from build123d import *

# Parameters (mm, degrees)
SKETCH1_R           = 15
SKETCH1_R_2         = 10
BOSS_EXTRUDE1_DEPTH = 125
SKETCH2_R           = 15
BOSS_EXTRUDE2_DEPTH = 40
SKETCH6_W           = 20
SKETCH6_H           = 5
BOSS_EXTRUDE6_DEPTH = 100
FILLET1_R           = 10
SKETCH8_W           = 28
SKETCH8_H           = 2
BOSS_EXTRUDE7_DEPTH = 30
CUT_EXTRUDE1_DEPTH  = 30
SKETCH10_R          = 6.25
CUT_EXTRUDE2_DEPTH  = 30


with BuildPart() as part:
    # Sketch1 → Boss-Extrude1 (new body)
    with BuildSketch(Plane(origin=(0, 0, 0), x_dir=(1, 0, 0), z_dir=(0, 1, 0))):
        with Locations(Location((0, 0, 0), (0, 0, 270))):
            Circle(SKETCH1_R)
        with Locations(Location((0, 0, 0), (0, 0, 270))):
            Circle(SKETCH1_R_2, mode=Mode.SUBTRACT)
    extrude(amount=BOSS_EXTRUDE1_DEPTH)

    # Sketch2 → Boss-Extrude2 (add)
    with BuildSketch(Plane.XY):
        with Locations((0, 62.5)):
            Circle(SKETCH2_R)
    extrude(amount=BOSS_EXTRUDE2_DEPTH)

    # Sketch6 → Boss-Extrude6 (add)
    with BuildSketch(Plane(origin=(0, 0, 0), x_dir=(0, 0, -1), z_dir=(1, 0, 0))):
        with Locations((0, 62.5)):
            Rectangle(SKETCH6_W, SKETCH6_H)
    extrude(amount=BOSS_EXTRUDE6_DEPTH)

    # Fillet1
    fillet1_edges = [part.edges().sort_by_distance(p)[0] for p in [
        (100, 62.5, -10),
        (100, 62.5, 10),
    ]]
    fillet(fillet1_edges, radius=FILLET1_R - 0.0001)  # a hair under: the kernel refuses the full size

    # Sketch8 → Boss-Extrude7 (add)
    with BuildSketch(Plane(origin=(0, 65, 0), x_dir=(1, 0, 0), z_dir=(0, 1, 0))):
        with Locations((28.5, 0)):
            Rectangle(SKETCH8_W, SKETCH8_H)
    extrude(amount=BOSS_EXTRUDE7_DEPTH)

    # Sketch9 → Cut-Extrude1 (cut)
    with BuildSketch(Plane(origin=(0, 0, -1), x_dir=(-1, 0, 0), z_dir=(0, 0, -1))):
        Polygon((-14.966629547, 95), (-42.5, 65), (-42.5, 95), align=None)
    extrude(amount=-CUT_EXTRUDE1_DEPTH, mode=Mode.SUBTRACT)

    # Sketch10 → Cut-Extrude2 (cut)
    with BuildSketch(Plane(origin=(0, 65, 0), x_dir=(1, 0, 0), z_dir=(0, 1, 0))):
        with Locations(Location((90, 0, 0), (0, 0, 270))):
            Circle(SKETCH10_R)
    extrude(amount=-CUT_EXTRUDE2_DEPTH, mode=Mode.SUBTRACT)


solid = part.part
Read the model definition and answer for the solid it produces. Units are mm, in the model's axes. A direction names the side the tool comes from. Give positions to 0.01 mm unless a question says otherwise; leave off trailing zeros. Write each loop counter-clockwise with the first axis right and the second up, starting at its lowest first coordinate (ties: lowest second). Pieces come first, ordered by that corner, then holes. Notation, with made-up numbers: (50.5, 22) - (108.5, 22) arc R27 ccw to (108.5, 56) - close; hole circle Ø4 at (6.5, -0.75). An arc over 180 degrees is marked (long way). Use CSV: the item, a comma, the result in double quotes. Start each with the question number.
Item 1: The part is cut by section B-B, the plane x = -8. Give the vertices of the cut face in (y, z).
Item 2: For faces 4 (the flat face through (4, 60, -4)), 5 (the flat face through (25, 76, 1)), 6 (the flat face through (55, 65, 0)), 7 (the cylindrical face through (-14.985, 63.16, 24.164)), determine the directions among +Z, -Z, +X, -X, +Y, -Y from which every point of the face is accessible in a straight line to the end or side of a thin tool.
Item 3: The part is cut by section D-D, the plane y = 97.5. Give the vertices of the cut face in (x, z).
Item 4: Consider line 1 (X direction, y = 37.5, z = 0); line 2 (Y direction, x = 44, z = 3.5); line 3 (X direction, y = 89.5, z = 0). Determine where each line is inside the solid, lowest interval first.
Item 5: The part is cut by section A-A, the plane y = 62.5. Count the separate pieces of the cut face and the enclosed holes in it, and give its area (3 significant figures).
Item 6: Flat-ended cylindrical pins translate along their axes: P1, Ø14, axis at x = 26, y = 81, coming from the +Z side; P2, Ø14, axis at x = 28.5, y = 86.5, coming from the -Z side; P3, Ø1.5, axis at x = 16.5, z = -0.5, coming from the +Y side; P4, Ø1, axis at x = 82, y = 58.5, coming from the -Z side. Find the tip coordinate at first contact, or state that the pin passes through.
Item 7: The part is cut by section C-C, the plane z = 4. Give the vertices of the cut face in (x, y).
Item 8: The mould has two halves that part along Z. Classify faces 1 (the cylindrical face through (0.66, 61.625, -14.985)), 2 (the flat face through (55, 60, 0)), 3 (the cylindrical face through (-0.2, 47.5, 3.8)): pulls with the +Z half, pulls with the -Z half, needs draft (parallel to the pull), parting line crosses it, or undercut.
Taken from the geometry:
1,outline,"(0, -12.69) - (125, -12.69) - (125, -6) - (0, -6) - close; (0, 6) - (49.81, 6) - (49.81, 0) - (75.19, 0) - (75.19, 6) - (125, 6) - (125, 12.69) - (75.19, 12.69) - (75.19, 40) - (49.81, 40) - (49.81, 12.69) - (0, 12.69) - close"
2,face 4,"-Y"
2,face 5,"+Z, +X, +Y"
2,face 6,"+X, +Y"
2,face 7,"+Z"
3,outline,"circle Ø30 at (0, 0); hole circle Ø20 at (0, 0)"
4,line 1,"-15 to -10, 10 to 15"
4,line 2,"60 to 65"
4,line 3,"-15 to -10, 10 to 20.01"
5,separate pieces,"1"
5,enclosed holes,"2"
5,area,"3,020 mm2"
6,P1,"z = 1"
6,P2,"z = -1"
6,P3,"y = 94.15"
6,P4,"through"
7,outline,"(-14.46, 0) - (-9.17, 0) - (-9.17, 50.63) arc R15 ccw to (9.17, 50.63) - (9.17, 0) - (14.46, 0) - (14.46, 58.5) arc R15 ccw to (14.79, 60) - (85.2, 60) - (85.2, 65) - (14.79, 65) arc R15 ccw to (14.46, 66.5) - (14.46, 125) - (9.17, 125) - (9.17, 74.37) arc R15 ccw to (-9.17, 74.37) - (-9.17, 125) - (-14.46, 125) - (-14.46, 66.5) arc R15 ccw to (-14.46, 58.5) - close; (94.8, 60) - (99.17, 60) - (99.17, 65) - (94.8, 65) - close"
8,face 1,"parting line crosses it"
8,face 2,"needs draft"
8,face 3,"undercut"
